Can you work these out from the model? Positions are in its coordinate system, mm. A direction names the side the tool comes from. Give positions to 0.01 mm unless a question says otherwise; leave off trailing zeros. Order: outer loops, then holes, each group sorted by start corner. A loop starts at its lowest first (then second) coordinate and runs counter-clockwise, first axis right, second up. Notation, with made-up numbers: (12, 44) - (18, 44) arc R26 ccw to (18, 63) - close; hole circle Ø1 at (0, 37.25). An arc over 180 degrees is marked (long way). Return JSON: item names as keys, results as strings.
```python
from build123d import *

# Parameters (mm, degrees)
F0_R     = 1.5
F0_R_2   = 4
F1_DEPTH = 4


# Not quite as in the source:
# - ends of sketch curves that miss each other by under 0.0002 mm in the source are joined


with BuildPart() as f1:
    # F0 (on Front) → F1 (new body)
    with BuildSketch(Plane.XZ):
        with BuildLine():
            ThreePointArc((-46.7520374748, 33.7019691352), (-47.1985525616, 33.1188473182), (-47.9229891353, 32.9980233677))
            ThreePointArc((-47.9229891353, 32.9980233677), (-48.7034151976, 32.8409436846), (-49.1218329373, 32.1636949909))
            ThreePointArc((-49.1218329373, 32.1636949909), (-49.0191167234, 26.9485703376), (-47.2444231086, 22.0436199391))
            ThreePointArc((-47.2444231086, 22.0436199391), (-46.9316892388, 21.5893722277), (-46.5410881725, 21.2000467918))
            ThreePointArc((-46.5410881725, 21.2000467918), (-45.835088561, 20.6717193883), (-45.0805279455, 20.2154261011))
            ThreePointArc((-45.0805279455, 20.2154261011), (-45.0596673609, 20.2042820611), (-45.0387197194, 20.1933025406))
            Line((-45.0387197194, 20.1933025406), (-34.428702, 14.685356))
            ThreePointArc((-34.428702, 14.685356), (-30.7249663127, 13.3838083991), (-26.831855016, 12.8784683528))
            Line((-26.831855016, 12.8784683528), (-18.940113, 12.75863))
            ThreePointArc((-18.940113, 12.75863), (-14.3281771728, 11.5292251091), (-10.0737090286, 9.3656889559))
            Line((-10.0737090286, 9.3656889559), (23.742856, -8.189399))
            ThreePointArc((23.742856, -8.189399), (26.6741197813, -10.1115239367), (29.157366832, -12.5854591375))
            ThreePointArc((29.157366832, -12.5854591375), (29.9965212655, -14.0706922033), (30.287531, -15.751588))
            Line((30.287531, -15.751588), (30.287531, -29.049112))
            ThreePointArc((30.287531, -29.049112), (30.0678610859, -29.5794420859), (29.537531, -29.799112))
            Line((29.537531, -29.799112), (28.787531, -29.799112))
            Line((28.787531, -29.799112), (28.787531, -31.799112))
            Line((28.787531, -31.799112), (29.537531, -31.799112))
            ThreePointArc((29.537531, -31.799112), (30.0678610859, -32.0187819141), (30.287531, -32.549112))
            Line((30.287531, -32.549112), (30.287531, -33.549112))
            ThreePointArc((30.287531, -33.549112), (30.5072009141, -34.0794420859), (31.037531, -34.299112))
            ThreePointArc((31.037531, -34.299112), (31.5678610859, -34.5187819141), (31.787531, -35.049112))
            Line((31.787531, -35.049112), (31.787531, -45.799112))
            Line((31.787531, -45.799112), (40.287531, -45.799112))
            Line((40.287531, -45.799112), (40.287531, -17.549112))
            ThreePointArc((40.287531, -17.549112), (42.9235699693, -11.1851509693), (49.287531, -8.549112))
            Line((49.287531, -8.549112), (49.287531, 1.450888))
            ThreePointArc((49.287531, 1.450888), (45.4037577728, 1.6406387059), (41.5569790733, 2.2080833707))
            ThreePointArc((41.5569790733, 2.2080833707), (33.2204107171, 4.4808989987), (25.2886487268, 7.9089034738))
            Line((25.2886487268, 7.9089034738), (-3.162569, 22.678696))
            ThreePointArc((-3.162569, 22.678696), (-7.380174163, 24.9132414841), (-11.0394989374, 27.9776710605))
            Line((-11.0394989374, 27.9776710605), (-15.678673, 34.362967))
            ThreePointArc((-15.678673, 34.362967), (-18.332187349, 37.2561568684), (-21.5279068846, 39.5363022038))
            Line((-21.5279068846, 39.5363022038), (-32.137926, 45.044248))
            ThreePointArc((-32.137926, 45.044248), (-32.1589591581, 45.0550621571), (-32.1800770412, 45.0657099174))
            ThreePointArc((-32.1800770412, 45.0657099174), (-32.9874548739, 45.4202604433), (-33.8258020362, 45.693644867))
            ThreePointArc((-33.8258020362, 45.693644867), (-34.3689763365, 45.7890671015), (-34.9204399653, 45.7834476614))
            ThreePointArc((-34.9204399653, 45.7834476614), (-39.9164421929, 44.4291859973), (-44.218633855, 41.550781845))
            ThreePointArc((-44.218633855, 41.550781845), (-44.5354399962, 40.8204576148), (-44.2185063254, 40.090188652))
            ThreePointArc((-44.2185063254, 40.090188652), (-43.903802542, 39.4265860913), (-44.1273026907, 38.7269757472))
            ThreePointArc((-44.1273026907, 38.7269757472), (-45.6966868361, 36.3487212178), (-46.7520374748, 33.7019691352))
        make_face()
        with Locations((34.037531, -30.549112)):
            Circle(F0_R, mode=Mode.SUBTRACT)
        with Locations((40.287531, -4.049112)):
            Circle(F0_R, mode=Mode.SUBTRACT)
        with BuildLine():
            Line((-29.443172, 22.692668), (-28.872421, 20.889608))
            ThreePointArc((-28.872421, 20.889608), (-29.8498040801, 19.0068647531), (-31.7325472924, 19.984248224))
            Line((-31.7325472924, 19.984248224), (-32.303298, 21.787307))
            ThreePointArc((-32.303298, 21.787307), (-31.3259155182, 23.6700510575), (-29.443172, 22.692668))
        make_face(mode=Mode.SUBTRACT)
        with BuildLine():
            Line((-40.461853, 26.022633), (-42.264913, 25.451882))
            ThreePointArc((-42.264913, 25.451882), (-44.1476570575, 26.4292644818), (-43.1702740637, 28.3120082014))
            Line((-43.1702740637, 28.3120082014), (-41.367214, 28.882759))
            ThreePointArc((-41.367214, 28.882759), (-39.4844709425, 27.9053765182), (-40.461853, 26.022633))
        make_face(mode=Mode.SUBTRACT)
        with Locations((-33.28753, 29.866991)):
            Circle(F0_R_2, mode=Mode.SUBTRACT)
        with BuildLine():
            Line((-26.113207, 33.711349), (-24.310148, 34.2821))
            ThreePointArc((-24.310148, 34.2821), (-22.4274039425, 33.3047175182), (-23.4047869363, 31.4219737986))
            Line((-23.4047869363, 31.4219737986), (-25.207847, 30.851223))
            ThreePointArc((-25.207847, 30.851223), (-27.0905902014, 31.8286059363), (-26.113207, 33.711349))
        make_face(mode=Mode.SUBTRACT)
        with BuildLine():
            Line((-37.131889, 37.041314), (-37.70264, 38.844374))
            ThreePointArc((-37.70264, 38.844374), (-36.7252563743, 40.727117103), (-34.8425130864, 39.7497349727))
            Line((-34.8425130864, 39.7497349727), (-34.271762, 37.946675))
            ThreePointArc((-34.271762, 37.946675), (-35.2491456257, 36.063930897), (-37.131889, 37.041314))
        make_face(mode=Mode.SUBTRACT)
    extrude(amount=F1_DEPTH)


solid = f1.part
```
1. If I drill on L1, parallel to Z at x = -34, y = -2.6; L2, parallel to Z at x = -26, y = -0.2; L3, parallel to X at y = -2.7, z = -39.5, over which ranges is the centre line in solid material (lowest first)? Write a range as [from, to].
Checks:
{"L1": "[14.49, 25.93], [33.8, 45.74]", "L2": "[12.87, 30.82], [33.75, 41.86]", "L3": "[31.79, 40.29]"}
2. On a 3-axis mill with a long thin cutter (end or side, diameter ignored), from which of +Z, -Z, +X, -X, +Y, -Y can I reach the whole of each face in a straight line? I mean faces 4 (the face through (40.288, -2, -32)), 5 (the face through (-36.8, -2, 40.7)). Say none if no direction works.
Checks:
{"face 4": "-Z, +X, +Y, -Y", "face 5": "+Y, -Y"}
3. For pin 1 Ø1 at (y, z) = (-2, -19) entering from +X; pin 2 Ø1.5 at (x, y) = (29.5, -0.5) entering from +Z; pin 3 Ø1 at (y, z) = (-0.5, -11.5) entering from +X, each with a flat end and sliding along its axis, tell me the tip position at first contact or that it passes through.
Checks:
{"pin 1": "x = 40.29", "pin 2": "z = 6.25", "pin 3": "x = 43.11"}
4. Suppose I cut it at C-C (x = 43.5). List the corners of the cut face in (y, z) for me.
Checks:
{"outline": "(-4, -10.66) - (0, -10.66) - (0, 1.87) - (-4, 1.87) - close"}
5. Thinking about a two-plate mould opening in Z: for faces 1 (the face through (33.335, -1.972, 4.441)), 2 (the face through (32.847, -1.972, -31.462)), 3 (the face through (36, -2, -45.799)), which applies, +Z half, -Z half, draft (parallel to the pull), parting line (faces both ways), or undercut?
Checks:
{"face 1": "+Z half", "face 2": "undercut", "face 3": "-Z half"}
6. Suppose I cut it at B-B (y = -2.6). State how many separate pieces and enclosed holes the cut face has, plus the area to 3 significant figures.
Checks:
{"separate pieces": "1", "enclosed holes": "7", "area": "2,130 mm^2"}
7. Suppose I cut it at A-A (x = 4.5). List the corners of the cut face in (y, z) for me.
Checks:
{"outline": "(-4, 1.8) - (0, 1.8) - (0, 18.7) - (-4, 18.7) - close"}
